For this review, take the finished solid that the model builds, in its own axes (mm). Face numbers are marked on the shaded views. A direction names the side the tool comes from. Give positions to 0.01 mm unless a question says otherwise; leave off trailing zeros. Write each loop counter-clockwise with the first axis right and the second up, starting at its lowest first coordinate (ties: lowest second). Pieces come first, ordered by that corner, then holes. Notation, with made-up numbers: M 2,56.25 L 48,56.25 A23 ccw 48,67.25 Z; hole C -21.5,-37 d5. An arc over 180 degrees is marked long. Answer as a JSON object with one key per item and string values. Group by question number.
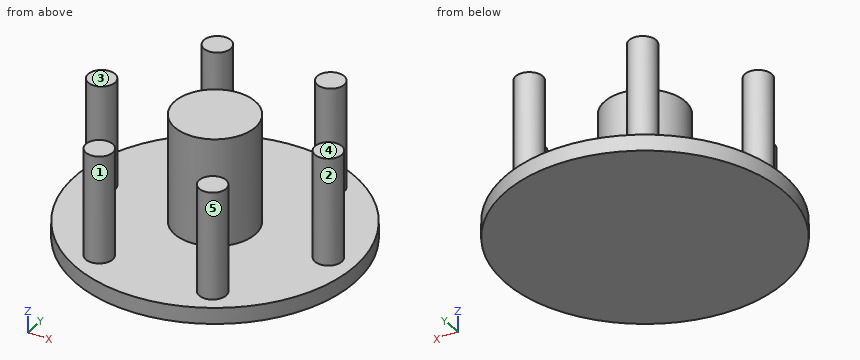
```python
from build123d import *

# Parameters (mm, degrees)
SKETCH_1_R      = 26
EXTRUDE_1_DEPTH = 3
SKETCH_2_R      = 2.5
EXTRUDE_2_DEPTH = 20
SKETCH_3_R      = 7.5
EXTRUDE_3_DEPTH = 20


with BuildPart() as part:
    # 草图1 → 凸台-拉伸1 (new body)
    with BuildSketch(Plane.XY):
        Circle(SKETCH_1_R)
    extrude(amount=-EXTRUDE_1_DEPTH)

    # 草图2 → 凸台-拉伸2 (add)
    with BuildSketch(Plane.XY):
        with Locations((-21, 0)):
            Circle(SKETCH_2_R)
        with Locations((-10.5, 18.186533479)):
            Circle(SKETCH_2_R)
        with Locations((10.5, 18.186533479)):
            Circle(SKETCH_2_R)
        with Locations((21, 0)):
            Circle(SKETCH_2_R)
        with Locations((10.5, -18.186533479)):
            Circle(SKETCH_2_R)
        with Locations((-10.5, -18.186533479)):
            Circle(SKETCH_2_R)
    extrude(amount=EXTRUDE_2_DEPTH)

    # 草图3 → 凸台-拉伸3 (add)
    with BuildSketch(Plane.XY):
        Circle(SKETCH_3_R)
    extrude(amount=EXTRUDE_3_DEPTH)


solid = part.part
```
Item 1: Consider section C-C (x = 0). Give the boundary of the cut face in (y, z), plus the area to 3 significant figures.
Item 2: Insertion check: P1, Ø8, axis at y = 18, z = 5, coming from the -X side; P2, Ø3, axis at x = -19.5, z = 2.5, coming from the -Y side; P3, Ø10, axis at x = -11, z = 17.5, coming from the -Y side. Each pin has a flat end and moves straight along its axis. Give the tip position at first contact, or say it passes through.
Item 3: Draft analysis for pull direction Y (two halves, no side actions). For the marked faces 1, 2 and 3, state which applies: released by +Y, released by -Y, zero draft, split by the parting line, or undercut.
Item 4: Machinability: for the marked faces 4 and 5, which of the approach directions +Z, -Z, +X, -X, +Y, -Y give a long, thin tool a straight path to every point of the face, cutting with its end or side? Answer none if there is none.
Item 5: Consider section B-B (y = 0). Give the boundary of the cut face in (x, z), plus the area to 3 significant figures.
Item 6: To check wall thickness, follow probe 1 along X at (y, z) = (-1, 4.5); probe 2 along X at (y, z) = (-0.5, 13.5); probe 3 along Z at (x, y) = (-16.5, -4). State the ranges of each line that lie inside material, in increasing order.
Item 7: Consider section D-D (x = -10.5). Give the boundary of the cut face in (y, z).
Item 8: Consider section A-A (z = 6.75). Give the boundary of the cut face in (x, y).
Result set:
{
 "1": {"outline": "M -26,-3 L 26,-3 L 26,0 L 7.5,0 L 7.5,20 L -7.5,20 L -7.5,0 L -26,0 Z", "area": "456 mm^2"},
 "2": {"P1": "stops at x = -13", "P2": "stops at y = -2.5", "P3": "stops at y = -20.69"},
 "3": {"face 1": "undercut", "face 2": "split by the parting line", "face 3": "zero draft"},
 "4": {"face 4": "+Z, +X, -X, +Y, -Y", "face 5": "+Z"},
 "5": {"outline": "M -26,-3 L 26,-3 L 26,0 L 23.5,0 L 23.5,20 L 18.5,20 L 18.5,0 L 7.5,0 L 7.5,20 L -7.5,20 L -7.5,0 L -18.5,0 L -18.5,20 L -23.5,20 L -23.5,0 L -26,0 Z", "area": "656 mm^2"},
 "6": {"probe 1": "x = -23.29 to -18.71, -7.43 to 7.43, 18.71 to 23.29", "probe 2": "x = -23.45 to -18.55, -7.48 to 7.48, 18.55 to 23.45", "probe 3": "z = -3 to 0"},
 "7": {"outline": "M -23.79,-3 L 23.79,-3 L 23.79,0 L 20.69,0 L 20.69,20 L 15.69,20 L 15.69,0 L -15.69,0 L -15.69,20 L -20.69,20 L -20.69,0 L -23.79,0 Z"},
 "8": {"outline": "C -21,0 d5; C -10.5,-18.19 d5; C -10.5,18.19 d5; C 0,0 d15; C 10.5,-18.19 d5; C 10.5,18.19 d5; C 21,0 d5"}
}
